Part model, mm, in its own coordinate system. Face numbers are marked on the shaded views. Round coordinates to 2 decimals unless told otherwise and drop trailing zeros. Order: outer loops, then holes, each group sorted by start corner. A loop starts at its lowest first (then second) coordinate and runs counter-clockwise, first axis right, second up. Notation, with made-up numbers: M 73.5,65 L 83.5,65 A32 cw 83.5,94 Z; hole C 2,34.25 d2. An arc over 180 degrees is marked long. Write each question's results on one line, items separated by ' | '. Start each with the question number.
1. Band-saw the part on D-D, the plane y = 30.5. List the corners of the cut face in (x, z).
2. Band-saw the part on A-A, the plane y = 43. List the corners of the cut face in (x, z), then the cut area to 3 significant figures.
3. Probe L1, parallel to Y at x = -51.5, z = 5; L2, parallel to Y at x = -44, z = 5; L3, parallel to Y at x = -14, z = 19. List the from-to ranges inside material, lowest first. Write a range as [from, to].
4. Band-saw the part on B-B, the plane y = 4. List the corners of the cut face in (x, z) (3 decimals), then the cut area to 4 significant figures.
5. Two-plate mould, pull along Z, no slides. Class the marked faces 1, 2 and 3: +Z half, -Z half, draft (parallel to the pull), parting line (faces both ways), or undercut.
6. Band-saw the part on C-C, the plane x = -43.5. List the corners of the cut face in (y, z).
7. Drop flat-ended pins along their axis: pin 1 Ø9 at (x, z) = (-14, 17) entering from +Y; pin 2 Ø10 at (x, y) = (-26, 6.5) entering from +Z; pin 3 Ø4 at (y, z) = (43, 3.35) entering from -X; pin 4 Ø9.5 at (x, z) = (-8.5, 17) entering from -Y. Give the stop position or say it passes through.
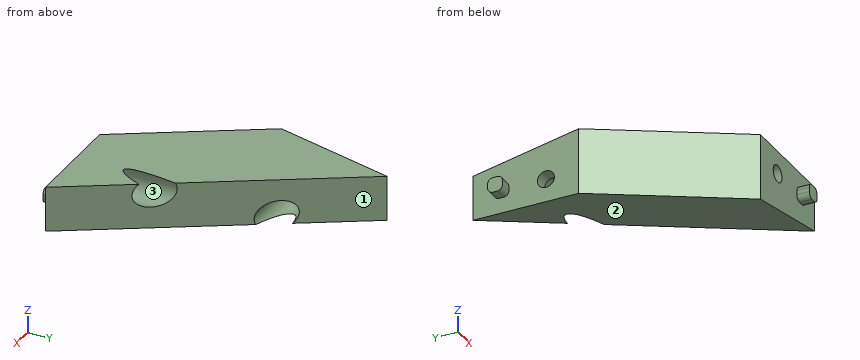
```python
from build123d import *

# Parameters (mm, degrees)
SKETCH2_W               = 63.5
SKETCH2_H               = 25.4
BOSS_EXTRUDE1_DEPTH     = 63.5
CUT_EXTRUDE1_DEPTH      = 90.356423253
SKETCH4_W               = 4.2
SKETCH4_H               = 4.2
BOSS_EXTRUDE2_DEPTH     = 3.5
SKETCH5_W               = 4.2
SKETCH5_H               = 4.2
BOSS_EXTRUDE3_DEPTH     = 3.5
FILLET1_R               = 1.5
CUT_EXTRUDE4_DEPTH      = 93.517057968
CUT_EXTRUDE5_DEPTH      = 91.824676174
SKETCH8_R               = 2.385
CUT_EXTRUDE6_DEPTH      = 94.305261385
CUT_EXTRUDE7_DEPTH      = 10
CUT_EXTRUDE7_DEPTH_BACK = 18
SKETCH12_R              = 4.2
SKETCH13_R              = 2.385
CUT_EXTRUDE8_DEPTH      = 95.953441302
CUT_EXTRUDE9_DEPTH      = 20
CUT_EXTRUDE9_DEPTH_BACK = 10
SKETCH14_R              = 4.2
SKETCH15_W              = 71.848813027
SKETCH15_H              = 26.708799916
CUT_EXTRUDE10_DEPTH     = 30


with BuildPart() as part:
    # Sketch2 → Boss-Extrude1 (new body)
    with BuildSketch(Plane(origin=(0, 0, 0), x_dir=(1, 0, 0), z_dir=(0, 1, 0))):
        with Locations((-25.757915773, -9.546483207)):
            Rectangle(SKETCH2_W, SKETCH2_H)
    extrude(amount=BOSS_EXTRUDE1_DEPTH)

    # Sketch3 → Cut-Extrude1 (cut, through all)
    with BuildSketch(Plane.XY.offset(22.246483207)):
        Polygon((-57.507915773, 63.5), (5.992084227, 0), (5.992084227, 63.5), align=None)
    extrude(amount=-CUT_EXTRUDE1_DEPTH, mode=Mode.SUBTRACT)

    # Sketch4 → Boss-Extrude2 (add)
    with BuildSketch(Plane.XZ):
        with Locations((-52.407915773, 15.746483207)):
            Rectangle(SKETCH4_W, SKETCH4_H)
        with Locations((-39.707915773, 15.746483207)):
            Rectangle(SKETCH4_W, SKETCH4_H)
        with Locations((-27.007915773, 15.746483207)):
            Rectangle(SKETCH4_W, SKETCH4_H)
        with Locations((-14.307915773, 15.746483207)):
            Rectangle(SKETCH4_W, SKETCH4_H)
        with Locations((-1.607915773, 15.746483207)):
            Rectangle(SKETCH4_W, SKETCH4_H)
    extrude(amount=BOSS_EXTRUDE2_DEPTH)

    # Sketch5 → Boss-Extrude3 (add)
    with BuildSketch(Plane.ZY.offset(57.507915773)):
        with Locations((3.346483207, 5.5)):
            Rectangle(SKETCH5_W, SKETCH5_H)
        with Locations((3.346483207, 18)):
            Rectangle(SKETCH5_W, SKETCH5_H)
        with Locations((3.346483207, 30.5)):
            Rectangle(SKETCH5_W, SKETCH5_H)
        with Locations((3.346483207, 43)):
            Rectangle(SKETCH5_W, SKETCH5_H)
        with Locations((3.346483207, 55.5)):
            Rectangle(SKETCH5_W, SKETCH5_H)
    extrude(amount=BOSS_EXTRUDE3_DEPTH)

    # Fillet1
    fillet1_edges = [part.edges().sort_by_distance(p)[0] for p in [
        (-59.257915773, 28.4, 1.246483207),
        (-59.257915773, 28.4, 5.446483207),
        (-59.257915773, 32.6, 5.446483207),
        (-59.257915773, 32.6, 1.246483207),
        (-59.257915773, 40.9, 1.246483207),
        (-59.257915773, 40.9, 5.446483207),
        (-59.257915773, 45.1, 5.446483207),
        (-59.257915773, 45.1, 1.246483207),
        (-59.257915773, 53.4, 1.246483207),
        (-59.257915773, 53.4, 5.446483207),
        (-59.257915773, 57.6, 5.446483207),
        (-59.257915773, 57.6, 1.246483207),
        (-54.507915773, -1.75, 17.846483207),
        (-54.507915773, -1.75, 13.646483207),
        (-50.307915773, -1.75, 13.646483207),
        (-50.307915773, -1.75, 17.846483207),
        (-37.607915773, -1.75, 17.846483207),
        (-41.807915773, -1.75, 17.846483207),
        (-41.807915773, -1.75, 13.646483207),
        (-37.607915773, -1.75, 13.646483207),
        (-24.907915773, -1.75, 17.846483207),
        (-29.107915773, -1.75, 17.846483207),
        (-29.107915773, -1.75, 13.646483207),
        (-24.907915773, -1.75, 13.646483207),
        (-12.207915773, -1.75, 17.846483207),
        (-16.407915773, -1.75, 17.846483207),
        (-16.407915773, -1.75, 13.646483207),
        (-12.207915773, -1.75, 13.646483207),
        (0.492084227, -1.75, 17.846483207),
        (-3.707915773, -1.75, 17.846483207),
        (-3.707915773, -1.75, 13.646483207),
        (0.492084227, -1.75, 13.646483207),
        (-59.257915773, 7.6, 1.246483207),
        (-59.257915773, 3.4, 1.246483207),
        (-59.257915773, 3.4, 5.446483207),
        (-59.257915773, 7.6, 5.446483207),
        (-59.257915773, 15.9, 1.246483207),
        (-59.257915773, 15.9, 5.446483207),
        (-59.257915773, 20.1, 5.446483207),
        (-59.257915773, 20.1, 1.246483207),
    ]]
    fillet(fillet1_edges, radius=FILLET1_R)

    # Sketch6 → Cut-Extrude4 (cut, through all)
    with BuildSketch(Plane.ZY.offset(57.507915773)):
        Polygon((22.246483207, 0), (9.546483207, 63.5), (22.246483207, 63.5), align=None)
    extrude(amount=-CUT_EXTRUDE4_DEPTH, mode=Mode.SUBTRACT)

    # Sketch7 → Cut-Extrude5 (cut, through all)
    with BuildSketch(Plane.XZ):
        Polygon((-57.507915773, -3.153516793), (5.992084227, 9.546483207), (5.992084227, -3.153516793), align=None)
    extrude(amount=-CUT_EXTRUDE5_DEPTH, mode=Mode.SUBTRACT)

    # Sketch8 → Cut-Extrude6 (cut, through all)
    with BuildSketch(Plane.XZ.offset(3.5)):
        with Locations(Location((-14.307915773, 15.746483207, 0), (0, 0, 270))):
            Circle(SKETCH8_R)
    extrude(amount=-CUT_EXTRUDE6_DEPTH, mode=Mode.SUBTRACT)

    # Sketch12 → Cut-Extrude7 (cut, two sides: drawn at the far end of the back side and taken through both)
    with BuildSketch(Plane(origin=(0, 23.204147495, 0), x_dir=(1, 0, 0), z_dir=(0, 1, 0)).offset(-CUT_EXTRUDE7_DEPTH_BACK)):
        with Locations(Location((-14.307915773, -15.746483207, 0), (0, 0, 203.417331866))):
            Circle(SKETCH12_R)
    extrude(amount=CUT_EXTRUDE7_DEPTH + CUT_EXTRUDE7_DEPTH_BACK, mode=Mode.SUBTRACT)

    # Sketch13 → Cut-Extrude8 (cut, through all)
    with BuildSketch(Plane.ZY.offset(61.007915773)):
        with Locations(Location((3.346483207, 43, 0), (0, 0, 200.648098404))):
            Circle(SKETCH13_R)
    extrude(amount=-CUT_EXTRUDE8_DEPTH, mode=Mode.SUBTRACT)

    # Sketch14 → Cut-Extrude9 (cut, two sides: drawn at the far end of the back side and taken through both)
    with BuildSketch(Plane.ZY.offset(33.553145543).offset(-CUT_EXTRUDE9_DEPTH_BACK)):
        with Locations(Location((3.346483207, 43, 0), (0, 0, 135.388680518))):
            Circle(SKETCH14_R)
    extrude(amount=CUT_EXTRUDE9_DEPTH + CUT_EXTRUDE9_DEPTH_BACK, mode=Mode.SUBTRACT)

    # Sketch15 → Cut-Extrude10 (cut)
    with BuildSketch(Plane(origin=(-11.853200292, -11.853200292, 0), x_dir=(0.7071067811865475, -0.7071067811865477, 0), z_dir=(0.7071067811865477, 0.7071067811865475, 0))):
        with Locations((-41.881900269, -9.453152274)):
            Rectangle(SKETCH15_W, SKETCH15_H)
    extrude(amount=-CUT_EXTRUDE10_DEPTH, mode=Mode.SUBTRACT)


solid = part.part
```
Solution:
1) outline: M -54.21,-2.49 L -24.51,3.45 L -24.51,16.15 L -54.21,16.15 Z
2) outline: M -57.51,-3.15 L -46.01,-0.85 L -53.55,-0.85 L -53.55,0.96 L -57.51,0.96 Z; M -57.51,5.73 L -53.55,5.73 L -53.55,7.55 L -37.01,7.55 L -37.01,13.65 L -57.51,13.65 Z | area: 153 mm^2
3) L1: [27.79, 39.14], [46.86, 57.49] | L2: [20.29, 39.14], [46.86, 49.99] | L3: [0, 5.2]
4) outline: M -27.706,2.807 L 1.992,8.746 L 1.992,21.446 L -27.706,21.446 Z; hole C -14.308,15.746 d4.77 | area: 447.5 mm^2
5) face 1: draft | face 2: -Z half | face 3: undercut
6) outline: M 19.79,-0.35 L 41.01,-0.35 A4.2 cw long 44.99,-0.35 L 49.49,-0.35 L 49.49,12.35 L 19.79,18.29 Z
7) pin 1: y = 24.49 | pin 2: z = 21.94 | pin 3: through | pin 4: y = 0
